```python
from build123d import *
from OCP.BRepFilletAPI import BRepFilletAPI_MakeChamfer

# Parameters (mm, degrees)
SKIZZE1_W                       = 73.6
SKIZZE1_H                       = 81.6
AUFSATZ_LINEAR_AUSTRAGEN1_DEPTH = 1.6
SKIZZE2_W                       = 73.6
SKIZZE2_H                       = 81.6
SKIZZE2_W_2                     = 70.4
SKIZZE2_H_2                     = 78.4
AUFSATZ_LINEAR_AUSTRAGEN2_DEPTH = 1.2
SKIZZE3_W                       = 23
SKIZZE3_H                       = 4
SCHNITT_LINEAR_AUSTRAGEN1_DEPTH = 1.6
AUFSATZ_LINEAR_AUSTRAGEN3_DEPTH = 1
VERRUNDUNG1_R                   = 0.6
FASE1_SIZE                      = 0.6
FASE1_SIZE2                     = 1.286704152
VERRUNDUNG2_R                   = 2


with BuildPart() as part:
    # Skizze1 → Aufsatz-Linear austragen1 (new body)
    with BuildSketch(Plane(origin=(0, -0.2, 0), x_dir=(1, 0, 0), z_dir=(0, 1, 0))):
        with Locations((35, 39)):
            Rectangle(SKIZZE1_W, SKIZZE1_H)
    extrude(amount=-AUFSATZ_LINEAR_AUSTRAGEN1_DEPTH)

    # Skizze2 → Aufsatz-Linear austragen2 (add)
    with BuildSketch(Plane(origin=(0, -0.2, 0), x_dir=(1, 0, 0), z_dir=(0, 1, 0))):
        with Locations((35, 39)):
            Rectangle(SKIZZE2_W, SKIZZE2_H)
        with Locations((35, 39)):
            Rectangle(SKIZZE2_W_2, SKIZZE2_H_2, mode=Mode.SUBTRACT)
    extrude(amount=AUFSATZ_LINEAR_AUSTRAGEN2_DEPTH)

    # Skizze3 → Schnitt-Linear austragen1 (cut)
    with BuildSketch(Plane.XY.offset(-78.2)):
        with Locations((35, 1.8)):
            Rectangle(SKIZZE3_W, SKIZZE3_H)
    extrude(amount=-SCHNITT_LINEAR_AUSTRAGEN1_DEPTH, mode=Mode.SUBTRACT)

    # Skizze4 → Aufsatz-Linear austragen3 (add)
    with BuildSketch(Plane(origin=(-1.8, 0, 0), x_dir=(0, 0, -1), z_dir=(1, 0, 0))):
        Polygon((63.2, 0), (63.2, 7), (72.6, 7), (72.6, 0), (70.8, 0), (70.8, 5.2), (65, 5.2), (65, 0), align=None)
        Polygon((14.8, 7), (5.4, 7), (5.4, 0), (7.2, 0), (7.2, 5.2), (13, 5.2), (13, 0), (14.8, 0), align=None)
    aufsatz_linear_austragen3 = extrude(amount=AUFSATZ_LINEAR_AUSTRAGEN3_DEPTH)

    # Spiegeln1: Aufsatz-Linear austragen3 across plane
    add(aufsatz_linear_austragen3.mirror(Plane(origin=(35, 0, 0), x_dir=(0, 0, 1), z_dir=(1, 0, 0))))

    # Verrundung1
    verrundung1_edges = [part.edges().sort_by_distance(p)[0] for p in [
        (70.8, 1, -64.1),
        (70.8, 1, -71.7),
        (70.8, 1, -13.9),
        (70.8, 1, -6.3),
        (-0.8, 1, -71.7),
        (-0.8, 1, -64.1),
        (-0.8, 1, -6.3),
        (-0.8, 1, -13.9),
    ]]
    fillet(verrundung1_edges, radius=VERRUNDUNG1_R - 0.0001)  # a hair under: the kernel refuses the full size

    # Fase1: one chamfer whose edges measure the first distance from different faces: ONE call of the kernel's chamfer builder (chamfer() names one face for all edges)
    fase1_edges_1 = [part.edges().sort_by_distance(p)[0] for p in [
        (70.8, 7, -67.9),
    ]]
    fase1_side_1 = [part.faces().sort_by_distance(p)[0] for p in [
        (71.3, 7, -67.9),
    ]]
    fase1_edges_2 = [part.edges().sort_by_distance(p)[0] for p in [
        (70.8, 7, -10.1),
    ]]
    fase1_side_2 = [part.faces().sort_by_distance(p)[0] for p in [
        (71.3, 7, -10.1),
    ]]
    fase1_edges_3 = [part.edges().sort_by_distance(p)[0] for p in [
        (-0.8, 7, -67.9),
    ]]
    fase1_side_3 = [part.faces().sort_by_distance(p)[0] for p in [
        (-1.3, 7, -67.9),
    ]]
    fase1_edges_4 = [part.edges().sort_by_distance(p)[0] for p in [
        (-0.8, 7, -10.1),
    ]]
    fase1_side_4 = [part.faces().sort_by_distance(p)[0] for p in [
        (-1.3, 7, -10.1),
    ]]
    fase1 = BRepFilletAPI_MakeChamfer(part.part.solid().wrapped)
    for e in fase1_edges_1:
        fase1.Add(FASE1_SIZE, FASE1_SIZE2, e.wrapped, fase1_side_1[0].wrapped)  # the first distance lies on this face
    for e in fase1_edges_2:
        fase1.Add(FASE1_SIZE, FASE1_SIZE2, e.wrapped, fase1_side_2[0].wrapped)  # the first distance lies on this face
    for e in fase1_edges_3:
        fase1.Add(FASE1_SIZE, FASE1_SIZE2, e.wrapped, fase1_side_3[0].wrapped)  # the first distance lies on this face
    for e in fase1_edges_4:
        fase1.Add(FASE1_SIZE, FASE1_SIZE2, e.wrapped, fase1_side_4[0].wrapped)  # the first distance lies on this face
    add(Compound.cast(fase1.Shape()), mode=Mode.REPLACE)

    # Verrundung2
    verrundung2_edges = [part.edges().sort_by_distance(p)[0] for p in [
        (-1.8, -0.4, -79.8),
        (71.8, -0.4, -79.8),
        (71.8, -0.4, 1.8),
        (-1.8, -0.4, 1.8),
    ]]
    fillet(verrundung2_edges, radius=VERRUNDUNG2_R)


solid = part.part
```
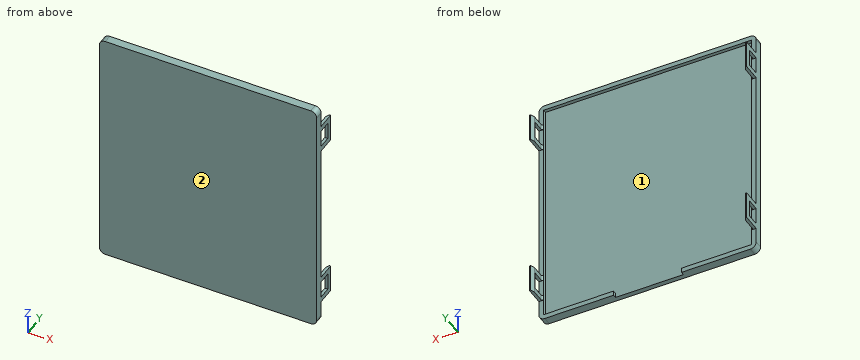
Geometry check sheet. Reference: the model listing, model coordinates, mm. Face numbers are marked on the shaded views. Round coordinates to 2 decimals unless told otherwise and drop trailing zeros. Order: outer loops, then holes, each group sorted by start corner. A loop starts at its lowest first (then second) coordinate and runs counter-clockwise, first axis right, second up. Notation, with made-up numbers: (79, 73.25) - (89, 73.25) arc R21 ccw to (89, 79.25) - close; hole circle Ø9 at (-23.75, 58.5). An arc over 180 degrees is marked (long way). Use a Markdown table: item, result. Add a question column.
(1) Sectioned sample at D-D, the plane x = 65. Enter the section's corners in (y, z).
(2) Sectioned sample at A-A, the plane z = -10. Enter the section's corners in (x, y), and give its area (3 significant figures).
(3) Sectioned sample at B-B, the plane y = 2.5. Count the separate pieces of the cut face and the enclosed holes in it, and give its area (3 significant figures).
(4) Depth check by flat-ended pin: pin 1 (1.3 mm diameter, centred on x = -1, y = 3.5, fed in from +Z); pin 2 (2 mm diameter, centred on x = 46, z = -29.5, fed in from +Y); pin 3 (0.5 mm diameter, centred on x = 71, y = 3.5, fed in from -Z). Enter the tip coordinate at first touch or a pass-through.
(5) Sectioned sample at C-C, the plane x = 24.5. Enter the section's corners in (y, z), and give its area (3 significant figures).
(6) Material ranges on line 1 along X through (y, z) = (0.5, -22.5); line 2 along Y through (x, z) = (62, -65); line 3 along Z through (x, y) = (48.5, 0.75), recorded low to high. Write a range as [from, to].
(7) Release check for a two-part mould opening along X. For the marked faces 1 and 2 record: pulls with the +X half, pulls with the -X half, needs draft (parallel to the pull), parting line crosses it, or undercut.
Answers below:
| question | item | result |
|---|---|---|
| 1 | outline | (-1.8, -79.8) - (1, -79.8) - (1, -78.2) - (-0.2, -78.2) - (-0.2, 0.2) - (1, 0.2) - (1, 1.8) - (-1.8, 1.8) - close |
| 2 | outline | (-1.8, -1.8) - (71.8, -1.8) - (71.8, 1) - (70.2, 1) - (70.2, -0.2) - (-0.2, -0.2) - (-0.2, 1) - (-1.8, 1) - close; (-1.8, 5.2) - (-0.8, 5.2) - (-0.8, 5.71) - (-1.4, 7) - (-1.8, 7) - close; (70.8, 5.2) - (71.8, 5.2) - (71.8, 7) - (71.4, 7) - (70.8, 5.71) - close |
| 2 | area | 124 mm² |
| 3 | separate pieces | 8 |
| 3 | enclosed holes | 0 |
| 3 | area | 14.4 mm² |
| 4 | pin 1 | z = -5.4 |
| 4 | pin 2 | y = -0.2 |
| 4 | pin 3 | z = -72.6 |
| 5 | outline | (-1.8, -79.8) - (-0.2, -79.8) - (-0.2, 0.2) - (1, 0.2) - (1, 1.8) - (-1.8, 1.8) - close |
| 5 | area | 132 mm² |
| 6 | line 1 | [-1.8, -0.2], [70.2, 71.8] |
| 6 | line 2 | [-1.8, -0.2] |
| 6 | line 3 | [-79.8, -78.2], [0.2, 1.8] |
| 7 | face 1 | undercut |
| 7 | face 2 | needs draft |
